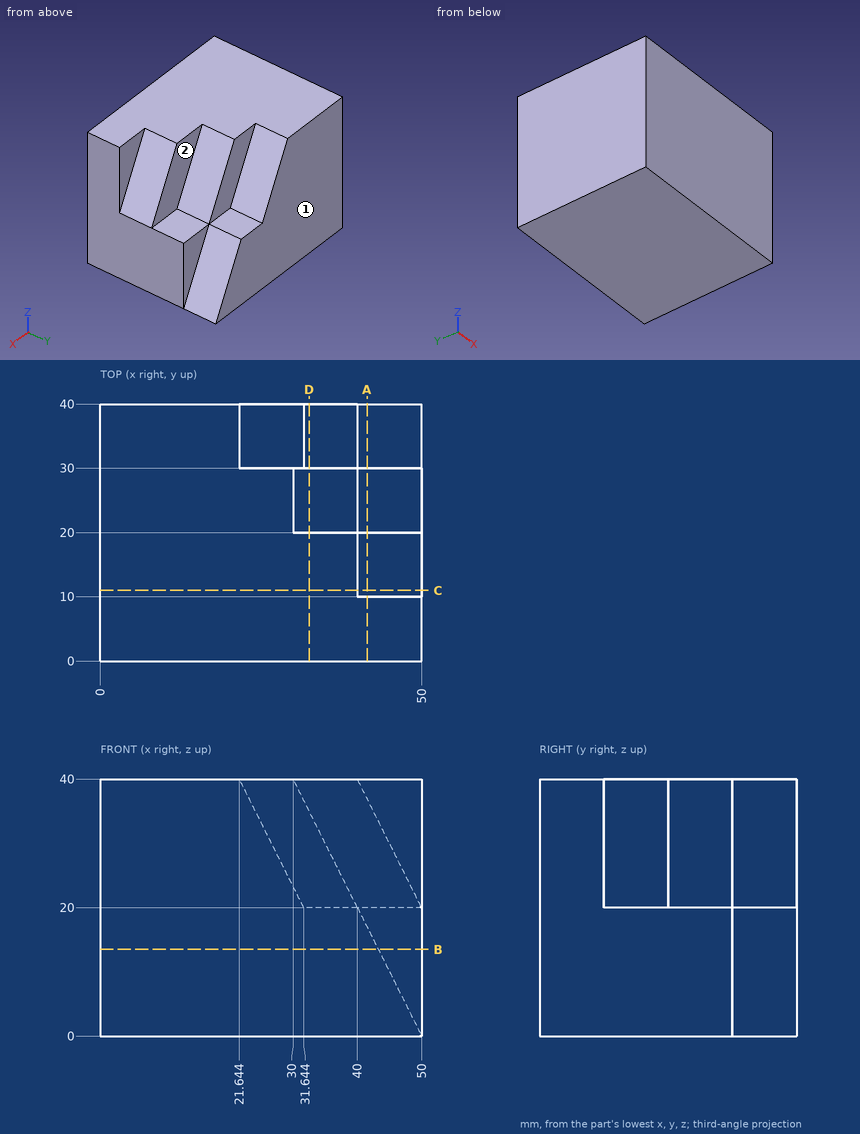
Print and shaded views of the part. All mm, measured from the part's lowest x, y and z. A direction names the side the tool comes from. Coordinates: 2 decimals unless noted, no trailing zeros. Write each loop counter-clockwise with the first axis right and the second up, starting at its lowest first coordinate (ties: lowest second). Pieces come first, ordered by that corner, then holes. Notation, with made-up numbers: M 3,14.5 L 50,14.5 A34 cw 50,46.5 Z; hole C 76.5,-19.75 d5. An arc over 180 degrees is marked long. Return JSON: item names as keys, results as strings.
1. Saw through at C-C, the plane y = 11. Write the cut outline in (x, z).
Determined:
{"outline": "M 0,0 L 50,0 L 50,20 L 40,40 L 0,40 Z"}
2. Probe L1, parallel to Y at x = 40, z = 25.5; L2, parallel to Y at x = 45, z = 37.5; L3, parallel to X at y = 21, z = 25. List the from-to ranges inside material, lowest first.
Determined:
{"L1": "0 to 20", "L2": "0 to 10", "L3": "0 to 37.5"}
3. 3-axis set-ups, long thin cutter, end or side, ignore diameter. For the marked faces 1 and 2: which of +Z, -Z, +X, -X, +Y, -Y reach the whole face in a straight line?
Determined:
{"face 1": "+Z, -Z, +X, -X, +Y", "face 2": "+Z, +X, +Y"}
4. Saw through at B-B, the plane z = 13.5. Write the cut outline in (x, y), then the cut area to 3 significant figures.
Determined:
{"outline": "M 0,0 L 50,0 L 50,30 L 43.25,30 L 43.25,40 L 0,40 Z", "area": "1,930 mm²"}
5. Saw through at A-A, the plane x = 41.5. Write the cut outline in (y, z), then the cut area to 3 significant figures.
Determined:
{"outline": "M 0,0 L 40,0 L 40,17 L 30,17 L 30,20 L 20,20 L 20,37 L 10,37 L 10,40 L 0,40 Z", "area": "1,140 mm²"}
6. Flat gauge pins, fed straight in: pin 1 Ø11 at (x, z) = (46.5, 28.5) entering from +Y; pin 2 Ø16 at (x, z) = (36.5, 34) entering from +Y; pin 3 Ø3 at (x, y) = (47, 24) entering from +Z. Where does each tip first touch, or does it go through?
Determined:
{"pin 1": "y = 20", "pin 2": "y = 30", "pin 3": "z = 20"}
7. Saw through at D-D, the plane x = 32.5. Write the cut outline in (y, z), then the cut area to 3 significant figures.
Determined:
{"outline": "M 0,0 L 40,0 L 40,20 L 30,20 L 30,35 L 20,35 L 20,40 L 0,40 Z", "area": "1,350 mm²"}
